Design review of the part built by this model. Coordinates are the model's own, in mm. Face numbers are marked on the shaded views. A direction names the side the tool comes from. Round coordinates to 2 decimals unless told otherwise and drop trailing zeros. Loops run counter-clockwise (first coordinate to the right, second up) from the corner with the lowest first, then second, coordinate; pieces in that order, holes last. Notation, with made-up numbers: M 35,58.25 L 51,58.25 A24 cw 51,89.25 Z; hole C 9.5,-35 d9. An arc over 180 degrees is marked long. Use a Markdown table: item, result.
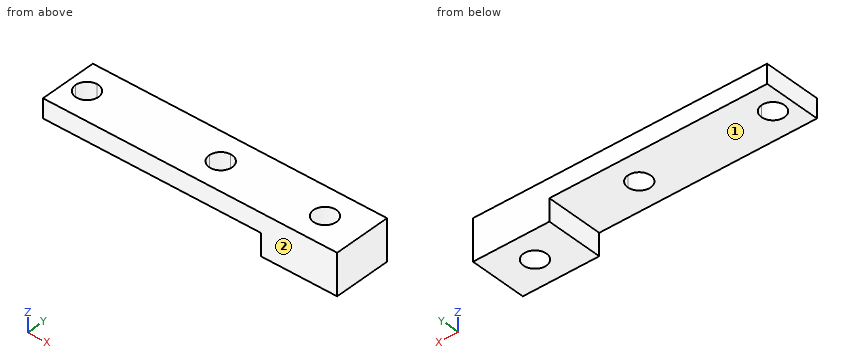
from build123d import *

# Parameters (mm, degrees)
BOSS_EXTRUDE1_DEPTH = 2.5
BOSS_EXTRUDE2_START = 2.9
SKETCH2_W           = 10
SKETCH2_H           = 7.5
SKETCH2_R           = 1.5
BOSS_EXTRUDE2_DEPTH = 2.9


with BuildPart() as part:
    # Sketch1 → Boss-Extrude1 (new body)
    with BuildSketch(Plane(origin=(0, 0, 0), x_dir=(0, 1, 0), z_dir=(0, 0, 1))):
        with BuildLine():
            Line((0, 18.25), (0, 19.25))
            Line((0, 19.25), (-3.75, 19.25))
            Line((-3.75, 19.25), (-3.75, -19.25))
            Line((-3.75, -19.25), (0, -19.25))
            Line((0, -19.25), (0, -15.898))
            ThreePointArc((0, -15.898), (-1.5, -14.398), (0, -12.898))
            Line((0, -12.898), (0, -2.25))
            ThreePointArc((0, -2.25), (-1.5, -0.75), (0, 0.75))
            Line((0, 0.75), (0, 15.25))
            ThreePointArc((0, 15.25), (-1.5, 16.75), (0, 18.25))
        make_face()
        with BuildLine():
            Line((3.75, 19.25), (0, 19.25))
            Line((0, 19.25), (0, 18.25))
            ThreePointArc((0, 18.25), (1.060660172, 17.810660172), (1.5, 16.75))
            ThreePointArc((1.5, 16.75), (1.060660172, 15.689339828), (0, 15.25))
            Line((0, 15.25), (0, 0.75))
            ThreePointArc((0, 0.75), (1.060660172, 0.310660172), (1.5, -0.75))
            ThreePointArc((1.5, -0.75), (1.060660172, -1.810660172), (0, -2.25))
            Line((0, -2.25), (0, -12.898))
            ThreePointArc((0, -12.898), (1.060660172, -13.337339828), (1.5, -14.398))
            ThreePointArc((1.5, -14.398), (1.060660172, -15.458660172), (0, -15.898))
            Line((0, -15.898), (0, -19.25))
            Line((0, -19.25), (3.75, -19.25))
            Line((3.75, -19.25), (3.75, 19.25))
        make_face()
    extrude(amount=BOSS_EXTRUDE1_DEPTH)

    # Sketch2 → Boss-Extrude2 (add)
    with BuildSketch(Plane(origin=(0, 0, 0), x_dir=(1, 0, 0), z_dir=(0, 0, -1)).offset(BOSS_EXTRUDE2_START)):
        with Locations((14.25, 0)):
            Rectangle(SKETCH2_W, SKETCH2_H)
        with Locations(Location((14.398, 0, 0), (0, 0, 180))):
            Circle(SKETCH2_R, mode=Mode.SUBTRACT)
    extrude(amount=-BOSS_EXTRUDE2_DEPTH)


solid = part.part
1. Insertion check: pin 1 (4 mm diameter, centred on x = 0, y = 1, fed in from -Z); pin 2 (2.5 mm diameter, centred on y = 1.5, z = -1.5, fed in from -X). Each pin has a flat end and moves straight along its axis. Give the tip position at first contact, or say it passes through.
Check values:
| item | result |
|---|---|
| pin 1 | stops at z = 0 |
| pin 2 | stops at x = 9.25 |
2. Take a section at B-B on z = 0.6. Give the boundary of the cut face in (x, y), and give its area (3 significant figures).
Check values:
| item | result |
|---|---|
| outline | M -19.25,-3.75 L 19.25,-3.75 L 19.25,3.75 L -19.25,3.75 Z; hole C -16.75,0 d3; hole C 0.75,0 d3; hole C 14.4,0 d3 |
| area | 268 mm² |
3. Take a section at A-A on y = 1. Give the boundary of the cut face in (x, z).
Check values:
| item | result |
|---|---|
| outline | M -19.25,0 L -17.87,0 L -17.87,2.5 L -19.25,2.5 Z; M -15.63,0 L -0.37,0 L -0.37,2.5 L -15.63,2.5 Z; M 1.87,0 L 9.25,0 L 9.25,-2.9 L 13.28,-2.9 L 13.28,2.5 L 1.87,2.5 Z; M 15.52,-2.9 L 19.25,-2.9 L 19.25,2.5 L 15.52,2.5 Z |
4. Take a section at C-C on z = -1.8. Give the boundary of the cut face in (x, y), and give its area (3 significant figures).
Check values:
| item | result |
|---|---|
| outline | M 9.25,-3.75 L 19.25,-3.75 L 19.25,3.75 L 9.25,3.75 Z; hole C 14.4,0 d3 |
| area | 67.9 mm² |
5. Take a section at D-D on x = -3.5. Give the boundary of the cut face in (y, z).
Check values:
| item | result |
|---|---|
| outline | M -3.75,0 L 3.75,0 L 3.75,2.5 L -3.75,2.5 Z |
6. Machinability: for the marked faces 1 and 2, which of the approach directions +Z, -Z, +X, -X, +Y, -Y give a long, thin tool a straight path to every point of the face, cutting with its end or side? Answer none if there is none.
Check values:
| item | result |
|---|---|
| face 1 | -Z, -X, +Y, -Y |
| face 2 | +Z, -Z, +X, -X, -Y |
7. Wall thickness on line 1 along X through (y, z) = (0.5, 0.6); line 2 along X through (y, z) = (0, -0.3); line 3 along Z through (x, y) = (-6.5, 1.5): over which ranges is each line inside the solid? List them lowest first. Write a range as from..to.
Check values:
| item | result |
|---|---|
| line 1 | x = -19.25..-18.16, -15.34..-0.66, 2.16..12.98, 15.81..19.25 |
| line 2 | x = 9.25..12.9, 15.9..19.25 |
| line 3 | z = 0..2.5 |
